Can you work these out from the model? Positions are in its coordinate system, mm. Face numbers are marked on the shaded views. A direction names the side the tool comes from. Coordinates: 2 decimals unless noted, no trailing zeros. Loops run counter-clockwise (first coordinate to the right, second up) from the corner with the lowest first, then second, coordinate; pieces in that order, holes last.
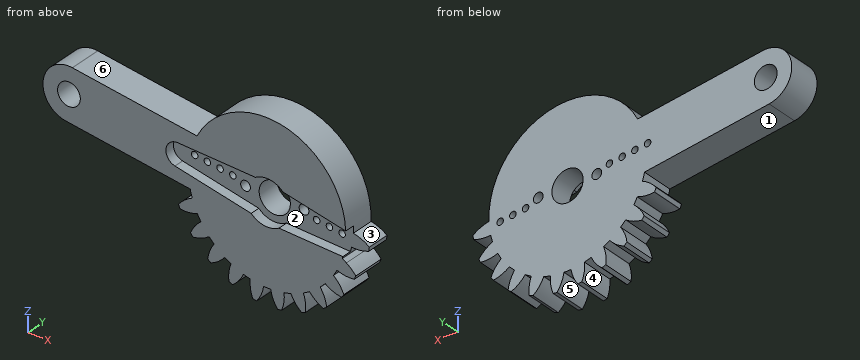
```python
from build123d import *

# Parameters (mm, degrees)
SKETCH1_R           = 1.75
SKETCH1_R_2         = 2.4
SKETCH1_R_3         = 0.75
BOSS_EXTRUDE1_DEPTH = 5
SKETCH2_R           = 0.500000007
SKETCH2_R_2         = 2.25
CUT_EXTRUDE1_DEPTH  = 48.168776066
CUT_EXTRUDE2_DEPTH  = 1.5


with BuildPart() as part:
    # Sketch1 → Boss-Extrude1 (new body)
    with BuildSketch(Plane(origin=(0, 4, 0), x_dir=(1, 0, 0), z_dir=(0, 1, 0))):
        with BuildLine():
            Line((1.43808022, 3.600125745), (2.081641936, 4))
            ThreePointArc((2.081641936, 4), (2.861028333, 4.588201733), (3.521749436, 5.30713988))
            ThreePointArc((3.521749436, 5.30713988), (3.405395609, 5.596745198), (3.282888305, 5.883801663))
            ThreePointArc((3.282888305, 5.883801663), (1.93527598, 5.894040025), (0.627094961, 5.57027124))
            ThreePointArc((0.627094961, 5.57027124), (0.366286148, 6.046375), (0.084372603, 6.510293938))
            ThreePointArc((0.084372603, 6.510293938), (1.018855105, 7.48132754), (1.683794586, 8.65351323))
            ThreePointArc((1.683794586, 8.65351323), (1.496450048, 8.903135899), (1.303821399, 9.148703928))
            ThreePointArc((1.303821399, 9.148703928), (-0.000522033, 8.809805691), (-1.180330337, 8.158486898))
            ThreePointArc((-1.180330337, 8.158486898), (-1.555477026, 8.550865528), (-1.947855656, 8.926012217))
            ThreePointArc((-1.947855656, 8.926012217), (-1.296536862, 10.105820521), (-0.957638625, 11.410163953))
            ThreePointArc((-0.957638625, 11.410163953), (-1.203206655, 11.602792602), (-1.452829324, 11.79013714))
            ThreePointArc((-1.452829324, 11.79013714), (-2.625015014, 11.125197659), (-3.596048616, 10.190715157))
            ThreePointArc((-3.596048616, 10.190715157), (-4.059967554, 10.472628702), (-4.536071314, 10.733437515))
            ThreePointArc((-4.536071314, 10.733437515), (-4.212302529, 12.041618533), (-4.222540891, 13.389230859))
            ThreePointArc((-4.222540891, 13.389230859), (-4.509597355, 13.511738163), (-4.799202674, 13.62809199))
            ThreePointArc((-4.799202674, 13.62809199), (-5.759348103, 12.682425791), (-6.455432668, 11.528463019))
            ThreePointArc((-6.455432668, 11.528463019), (-6.976508546, 11.680699536), (-7.503891752, 11.809396783))
            ThreePointArc((-7.503891752, 11.809396783), (-7.529737283, 13.156800143), (-7.888414517, 14.455843809))
            ThreePointArc((-7.888414517, 14.455843809), (-8.197396993, 14.499881098), (-8.507248835, 14.537314892))
            ThreePointArc((-8.507248835, 14.537314892), (-9.18992168, 13.375367565), (-9.563620196, 12.080565177))
            ThreePointArc((-9.563620196, 12.080565177), (-10.106342554, 12.09275), (-10.649064912, 12.080565177))
            ThreePointArc((-10.649064912, 12.080565177), (-11.022763428, 13.375367565), (-11.705436272, 14.537314892))
            ThreePointArc((-11.705436272, 14.537314892), (-12.015288115, 14.499881098), (-12.324270591, 14.455843809))
            ThreePointArc((-12.324270591, 14.455843809), (-12.682947825, 13.156800143), (-12.708793355, 11.809396783))
            ThreePointArc((-12.708793355, 11.809396783), (-13.236176561, 11.680699536), (-13.757252439, 11.528463019))
            ThreePointArc((-13.757252439, 11.528463019), (-14.453337005, 12.682425791), (-15.413482434, 13.62809199))
            ThreePointArc((-15.413482434, 13.62809199), (-15.703087752, 13.511738163), (-15.990144217, 13.389230859))
            ThreePointArc((-15.990144217, 13.389230859), (-16.000382579, 12.041618533), (-15.676613793, 10.733437515))
            ThreePointArc((-15.676613793, 10.733437515), (-16.152717554, 10.472628702), (-16.616636492, 10.190715157))
            ThreePointArc((-16.616636492, 10.190715157), (-17.587670094, 11.125197659), (-18.759855783, 11.79013714))
            ThreePointArc((-18.759855783, 11.79013714), (-19.009478453, 11.602792602), (-19.255046482, 11.410163953))
            ThreePointArc((-19.255046482, 11.410163953), (-18.916148245, 10.105820521), (-18.264829452, 8.926012217))
            ThreePointArc((-18.264829452, 8.926012217), (-18.657208082, 8.550865528), (-19.032354771, 8.158486898))
            ThreePointArc((-19.032354771, 8.158486898), (-20.212163074, 8.809805691), (-21.516506507, 9.148703928))
            ThreePointArc((-21.516506507, 9.148703928), (-21.709135156, 8.903135899), (-21.896479694, 8.65351323))
            ThreePointArc((-21.896479694, 8.65351323), (-21.231540213, 7.48132754), (-20.297057711, 6.510293938))
            ThreePointArc((-20.297057711, 6.510293938), (-20.578971255, 6.046375), (-20.839780068, 5.57027124))
            ThreePointArc((-20.839780068, 5.57027124), (-22.147961087, 5.894040025), (-23.495573413, 5.883801663))
            ThreePointArc((-23.495573413, 5.883801663), (-23.618080717, 5.596745198), (-23.734434544, 5.30713988))
            ThreePointArc((-23.734434544, 5.30713988), (-22.788768345, 4.346994451), (-21.634805572, 3.650909885))
            ThreePointArc((-21.634805572, 3.650909885), (-21.803584999, 3.067429176), (-21.942853375, 2.47620963))
            Line((-21.942853375, 2.47620963), (-41.11537681, -0.047900965))
            ThreePointArc((-41.11537681, -0.047900965), (-44.559051487, -4.53578518), (-40.071167272, -7.979459856))
            Line((-40.071167272, -7.979459856), (-20.898643838, -5.455349261))
            ThreePointArc((-20.898643838, -5.455349261), (-7.038913378, -11.697242445), (1.974222624, 0.542722358))
            ThreePointArc((1.974222624, 0.542722358), (3.269025011, 0.916420874), (4.430972339, 1.599093719))
            ThreePointArc((4.430972339, 1.599093719), (4.393538544, 1.908945561), (4.349501255, 2.217928037))
            ThreePointArc((4.349501255, 2.217928037), (3.050457589, 2.576605271), (1.70305423, 2.602450802))
            ThreePointArc((1.70305423, 2.602450802), (1.581217534, 3.104116905), (1.43808022, 3.600125745))
        make_face()
        with Locations(Location((-40.593272041, -4.013680411, 0), (0, 0, 90))):
            Circle(SKETCH1_R, mode=Mode.SUBTRACT)
        with Locations(Location((-10.106342554, 0, 0), (0, 0, 90))):
            Circle(SKETCH1_R_2, mode=Mode.SUBTRACT)
        with Locations(Location((-5.606342554, 0, 0), (0, 0, 90))):
            Circle(SKETCH1_R_3, mode=Mode.SUBTRACT)
        with Locations(Location((-14.606342554, 0, 0), (0, 0, 90))):
            Circle(SKETCH1_R_3, mode=Mode.SUBTRACT)
    extrude(amount=-BOSS_EXTRUDE1_DEPTH)

    # Sketch2 → Cut-Extrude1 (cut, through all)
    with BuildSketch(Plane.XZ.offset(1)):
        with Locations(Location((-22.425502423, 1.456820148, 0), (0, 0, 270))):
            Circle(SKETCH2_R)
        with Locations(Location((-16.556398443, 0.76276073, 0), (0, 0, 270))):
            Circle(SKETCH2_R)
        with Locations(Location((-20.469134429, 1.225467009, 0), (0, 0, 270))):
            Circle(SKETCH2_R)
        with Locations(Location((-18.512766436, 0.994113869, 0), (0, 0, 270))):
            Circle(SKETCH2_R)
        with Locations(Location((-3.656286665, -0.76276073, 0), (0, 0, 270))):
            Circle(SKETCH2_R)
        with Locations(Location((-1.699918672, -0.994113869, 0), (0, 0, 270))):
            Circle(SKETCH2_R)
        with Locations(Location((0.256449322, -1.225467009, 0), (0, 0, 270))):
            Circle(SKETCH2_R)
        with Locations((-10.106342554, 0)):
            Circle(SKETCH2_R_2)
    extrude(amount=-CUT_EXTRUDE1_DEPTH, mode=Mode.SUBTRACT)

    # Sketch3 → Cut-Extrude2 (cut)
    with BuildSketch(Plane.XZ.offset(1)):
        with BuildLine():
            Line((4.066067931, 0.080576868), (-7.656447881, 2.429097794))
            ThreePointArc((-7.656447881, 2.429097794), (-9.701180965, 3.426126689), (-11.922071261, 2.933535284))
            Line((-11.922071261, 2.933535284), (-23.869034652, 3.384083008))
            ThreePointArc((-23.869034652, 3.384083008), (-25.672874683, 1.840842872), (-24.278753039, -0.080576868))
            Line((-24.278753039, -0.080576868), (-12.556237227, -2.429097794))
            ThreePointArc((-12.556237227, -2.429097794), (-10.511504143, -3.426126689), (-8.290613847, -2.933535284))
            Line((-8.290613847, -2.933535284), (3.656349544, -3.384083008))
            ThreePointArc((3.656349544, -3.384083008), (5.460189575, -1.840842872), (4.066067931, 0.080576868))
        make_face()
    extrude(amount=-CUT_EXTRUDE2_DEPTH, mode=Mode.SUBTRACT)


solid = part.part
```
Item 1: Suppose I cut it at C-C, the plane x = -29.5. Please give me the cut outline in (y, z), plus the area to 3 significant figures.
Results are:
outline: (-1, -1.48) - (4, -1.48) - (4, 6.59) - (-1, 6.59) - close
area: 40.3 mm2
Item 2: Suppose I cut it at A-A, the plane z = 4.75. Please give me the cut outline in (x, y), plus the area to 3 significant figures.
Results are:
outline: (-44.52, -1) - (-42.18, -1) - (-42.18, 4) - (-44.52, 4) - close; (-39.01, -1) - (1.01, -1) - (1.01, 4) - (-39.01, 4) - close
area: 212 mm2
Item 3: We'd pull the mould along X, two halves only. Please class the marked faces 1, 2 and 3: +X half, -X half, draft (parallel to the pull), parting line (faces both ways), or undercut.
Results are:
face 1: -X half
face 2: undercut
face 3: +X half
Item 4: On a 3-axis mill with a long thin cutter (end or side, diameter ignored), from which of +Z, -Z, +X, -X, +Y, -Y can I reach the whole of each face in a straight line? I mean the marked faces 4, 5 and 6. Say none if no direction works.
Results are:
face 4: +Y, -Y
face 5: -Z, +Y, -Y
face 6: +Z, +Y, -Y
Item 5: Suppose I cut it at B-B, the plane y = 1.95. Count the separate pieces of the cut face and the enclosed holes in it, plus the area to 3 significant figures.
Results are:
separate pieces: 1
enclosed holes: 11
area: 643 mm2
Item 6: I'm going to push flat-ended pins straight in: P1, Ø1.5, axis at y = 1.5, z = 7, coming from the +X side; P2, Ø1.2, axis at x = -22.43, z = 1.46, coming from the -Y side; P3, Ø0.6, axis at x = -18.51, z = 0.99, coming from the +Y side; P4, Ø1.3, axis at x = -20.47, z = 1.23, coming from the +Y side. Where does each tip first touch, or does it pass through?
Results are:
P1: stops at x = 0.25
P2: stops at y = 0.5
P3: passes through
P4: stops at y = 4
Item 7: I need wall thicknesses on line 1 along X through (y, z) = (1.85, -8.25); line 2 along Z through (x, y) = (-21.5, -0.25); line 3 along Y through (x, z) = (-5, -3). Which ranges of each line are inside material? Lowest first, please.
Results are:
line 1: x = -21.71 to -19.16, -18.95 to -1.26, -1.05 to 1.5
line 2: z = -9.15 to -7.88, -5.78 to -0.64, 3.29 to 5.53
line 3: y = 0.5 to 4
